Input: part model. Units: mm. Frame: model coordinates. A direction names the side the tool comes from. Give positions to 0.01 mm unless a question says otherwise; leave off trailing zeros. Write each loop counter-clockwise with the first axis right and the second up, starting at its lowest first coordinate (ties: lowest second). Pieces come first, ordered by that corner, then holes.
```python
from build123d import *

# Parameters (mm, degrees)
F3_W     = 10
F3_H     = 4.6456689391
F4_DEPTH = 25
F5_R     = 1.5
F6_DEPTH = 4


with BuildPart() as f1:
    # F0 (on Front) → F1 (revolve)
    with BuildSketch(Plane.XZ):
        with BuildLine():
            Line((-2.3, 0), (2.3, 0))
            ThreePointArc((2.3, 0), (0, 2.3), (-2.3, 0))
        make_face()
    revolve(axis=Axis((0, 0, 0), (1, 0, 0)))

    # F3 (on offset) → F4 (cut)
    with BuildSketch(Plane.XZ.offset(10)):
        with Locations((0.6477613404, 2.3228344696)):
            Rectangle(F3_W, F3_H)
    extrude(amount=-F4_DEPTH, mode=Mode.SUBTRACT)

    # F5 (on face) → F6 (join)
    with BuildSketch(Plane.XY):
        with Locations((-0.1185681322, 0.0726561921)):
            Circle(F5_R)
    extrude(amount=F6_DEPTH)


solid = f1.part
```
Q1. Material intervals for line 1 along Y through (x, z) = (-0.1, 0.25); line 2 along Z through (x, y) = (0.3, -1.6); line 3 along Z through (x, y) = (-1.8, -0.3), sorted ascending.
Q2. Section D-D, the plane x = -1.8. Return the cut outline in (y, z), then the cut area to 3 significant figures.
Q3. Section A-A, the plane x = 0.85. Return the cut outline in (y, z), then the cut area to 3 significant figures.
Q4. Access query for faces 1 (the cylindrical face through (-0.4, -1.4, 2)), 2 (the flat face through (0, 0, 4)). Directions: +Z, -Z, +X, -X, +Y, -Y. A direction counts if a zero-diameter tool reaches every point of the face in a straight line with its end or side. Return the directions, or none.
Q5. Section C-C, the plane z = 3.25. Return the cut outline in (x, y).
Q6. Pin query (flat end, axial travel): pin 1 (1.5 mm diameter, centred on x = 0.5, z = 1.5, fed in from -Y); pin 2 (1 mm diameter, centred on x = 1.5, y = -1.5, fed in from +Z); pin 3 (1 mm diameter, centred on x = 1.5, y = 0.5, fed in from -Z). Return the tip coordinate at first contact, or that it passes through.
Q7. Section B-B, the plane y = 0.45. Return the cut outline in (x, z).
Solutions:
1. line 1: y = -1.43 to 1.57
1. line 2: z = -1.62 to 0
1. line 3: z = -1.4 to 0
2. outline: (-1.43, 0) arc R1.43 ccw to (1.43, 0) - close
2. area: 3.22 mm2
3. outline: (-2.14, 0) arc R2.14 ccw to (2.14, 0) - (1.22, 0) - (1.22, 4) - (-1.07, 4) - (-1.07, 0) - close
3. area: 16.3 mm2
4. face 1: +Z
4. face 2: +Z, +X, -X, +Y, -Y
5. outline: circle Ø3 at (-0.12, 0.07)
6. pin 1: stops at y = -1.43
6. pin 2: stops at z = 0
6. pin 3: stops at z = -2.03
7. outline: (-2.26, 0) arc R2.26 ccw to (2.26, 0) - (1.33, 0) - (1.33, 4) - (-1.57, 4) - (-1.57, 0) - close
